Autodesk Inventor part; units mm, degrees
ref_plane "Work Plane7" through (0, -46.7931, -140.1287) normal (0, -0.9797, 0.2004) x (0, -0.2004, -0.9797)
ref_plane "Work Plane8" through (0, 46.7931, -140.1287) normal (0, -0.9797, -0.2004) x (0, 0.2004, -0.9797)
ref_plane "Work Plane9" through (-30, 0, 0) normal (1, 0, 0) x (0, 1, 0)
sketch "Sketch17" plane through (0, 0, 0) normal (1, 0, 0) x (0, 1, 0)
  line L0 (-151.0923, 0) -> (102.6542, 0) construction
  line L1 (0, -220) -> (0, 200)
  circle A0 centre (0, 0) radius 40
  circle A1 centre (0, 0) radius 48.5
  arc A2 (-55.3685, -137.8628) -> (55.3685, -137.8628) centre (0, 54.3203) ccw
  arc A3 (-60, -153.9388) -> (60, -153.9388) centre (0, 140) ccw
  line L2 (55.3685, -137.8628) -> (60, -153.9388)
  line L3 (-60, -153.9388) -> (-55.3685, -137.8628)
  line L4 (-30, -38.1084) -> (-30, -145.6797)
  line L5 (-30, -145.6797) -> (30, -145.6797)
  line L6 (30, -145.6797) -> (30, -38.1084)
  line L7 (-46.7931, -140.1287) -> (-50, -155.804)
  line L8 (46.7931, -140.1287) -> (50, -155.804)
  line L9 (-50, -155.804) -> (-28.8985, -159.3708) construction
  line L10 (-46.7931, -140.1287) -> (-25.9862, -145.1357) construction
  line L11 (-48.3965, -147.9663) -> (-7.733, -156.2855) construction
  arc A4 (26.4209, -129.6797) -> (26, -145.6797) centre (66.4047, -138.7371) ccw
  arc A5 (26.4209, -129.6797) -> (30, -97.6797) centre (-114.8428, -97.6797) ccw
  point P0 (0, -160)
  point P1 (0, -145.6797)
  point P2 (0, -160)
  point P3 (0, -48.5)
  point P4 (0, -145.6797)
  dimension "d173" = 97
  dimension "d174" = 80
  dimension "d224" = 60
  dimension "d229" = 160
  dimension "d230" = 300
  dimension "d231" = 16.7299
  dimension "d232" = 100
  dimension "d233" = 10
  dimension "d235" = 200
  dimension "d241" = 16
  dimension "d242" = 16.7931
  dimension "d243" = 16
  dimension "d244" = 32
  dimension "d245" = 26
sketch "Sketch16" plane through (0, 0, 0) normal (1, 0, 0) x (0, 1, 0)
  circle A0 centre (0, 0) radius 40
  circle A1 centre (0, 0) radius 48.5
  line L0 (0, -201.7) -> (0, 90.2) construction
  line L1 (0, -160) -> (0, -48.5)
  line L2 (30, -38.1084) -> (30, -103.6436)
  line L3 (30, -103.6436) -> (25, -132)
  line L4 (25, -132) -> (50, -132)
  line L5 (50, -132) -> (50, -160)
  line L6 (50, -160) -> (0, -160)
  dimension "d156" = 97
  dimension "d157" = 80
  dimension "d202" = 28
  dimension "d203" = 60
  dimension "d204" = 50
  dimension "d206" = 160
  dimension "d209" = 50
  dimension "d210" = 80
  dimension "d211" = 28.7938
extrude "Extrusion14" [suppressed]
fillet "Fillet10" [suppressed]
mirror "Mirror1" [suppressed]
thicken "Thicken1" [suppressed]
sketch "Sketch19" plane through (0, 0, 0) normal (0, 1, 0) x (-1, 0, 0)
  arc A0 (-110.8458, -111.0605) -> (110.8458, -111.0605) centre (0, -10) ccw
  line L0 (155.1841, 0) -> (-155.1841, 0)
  line L1 (0, -264.129) -> (0, 44.0215)
  line L2 (110.8458, -111.0605) -> (110.8458, -220.1075)
  line L3 (110.8458, -220.1075) -> (-110.8458, -220.1075)
  line L4 (-110.8458, -220.1075) -> (-110.8458, -111.0605)
  point P0 (0, 0)
  point P1 (0, -160)
  point P2 (0, -160)
  point P3 (0, -220.1075)
  dimension "d217" = 150
  dimension "d218" = 0
revolve "Revolution1" [suppressed]
fillet "Fillet15" [suppressed]
revolve "Revolution2" add sketch "Sketch17" angle 360 about axis through (0, 0, -10) along (0, 0, 1) separate body contours L1 L5 L6 A2 L8 A3 | A2 A4 L5 | L8 A2 L2 A3 | A2 L6 L5 A4
ref_plane "Work Plane7" through (0, -46.7931, -140.1287) normal (0, -0.9797, 0.2004) x (0, -0.2004, -0.9797)
split "Split2" plane through (0, -46.7931, -140.1287) removes the side toward (0, -0.9797, 0.2004)
ref_plane "Work Plane8" through (0, 46.7931, -140.1287) normal (0, -0.9797, -0.2004) x (0, 0.2004, -0.9797)
split "Split3" plane through (0, 46.7931, -140.1287) removes the side toward (0, 0.9797, 0.2004)
ref_plane "Work Plane9" through (-30, 0, 0) normal (1, 0, 0) x (0, 1, 0)
split "Split4" plane through (-30, 0, 0) removes the side toward (-1, 0, 0)
ref_plane "Work Plane10" through (30, 0, 0) normal (1, 0, 0) x (0, 1, 0)
split "Split5" plane through (30, 0, 0) removes the side toward (1, 0, 0)
extrude "Extrusion17" add sketch "Sketch17" along normal mid plane 60 contours L1 A1 L6 A5 A4 A2 | A2 A4 L5 | A4 A5 L6 A2 | A2 L6 L5 A4
fillet "Fillet16" radius 5 1 edges at (0, 30, -38.1084)
mirror "Mirror4" about plane through (0, 0, 0) normal (0, 1, 0) of "Extrusion17", "Fillet16"
properties part number "shank_2"
Here's how the part is built. I have some questions about the finished solid (model axes, mm). Round coordinates to 2 decimals unless told otherwise and drop trailing zeros. Order: outer loops, then holes, each group sorted by start corner. A loop starts at its lowest first (then second) coordinate and runs counter-clockwise, first axis right, second up. Notation, with made-up numbers: M 49.5,34 L 54.5,34 A19 ccw 54.5,38 Z; hole C 0,21.5 d3. An arc over 180 degrees is marked long. Use CSV: the item, a comma, the result in double quotes.
1) If we mould it in two halves opening along Y, with no side actions, what happens to faces 1 (the flat face through (-30, -1, -100)), 2 (the cylindrical face through (-0.42, 27.52, -42.98)), 3 (the flat face through (-0.42, 48.144, -146.732))? For each: pulls with the +Y half, pulls with the -Y half, needs draft (parallel to the pull), parting line crosses it, or undercut.
Taken from the geometry:
face 1,"needs draft"
face 2,"undercut"
face 3,"pulls with the +Y half"
2) I want a section at A-A (x = 18). List the corners of the cut face in (y, z) for me, then the cut area to 3 significant figures.
Taken from the geometry:
outline,"M -49.89,-155.27 A299.46 ccw 49.89,-155.27 L 46.63,-139.33 A199.19 cw 30,-142.6 L 30,-47.3 A5 ccw 22.66,-42.88 A48.5 cw -22.66,-42.88 A5 ccw -30,-47.3 L -30,-142.6 A199.19 cw -46.63,-139.33 Z"
area,"7,370 mm^2"
3) I need wall thicknesses on line 1 along Y through (x, z) = (14.5, -94); line 2 along Z through (x, y) = (-12.5, -6); line 3 along Z through (x, y) = (5.5, 43). Which ranges of each line are inside material? Lowest first, please. Write a range as [from, to].
Taken from the geometry:
line 1,"[-30, 30]"
line 2,"[-159.68, -48.13]"
line 3,"[-156.85, -140.93]"
4) I want a section at B-B (z = -107.5). List the corners of the cut face in (x, y) for me.
Taken from the geometry:
outline,"M -30,-30 L 30,-30 L 30,30 L -30,30 Z"
5) I want a section at D-D (x = -17). List the corners of the cut face in (y, z) for me.
Taken from the geometry:
outline,"M -49.9,-155.33 A299.52 ccw 49.9,-155.33 L 46.65,-139.42 A199.28 cw 30,-142.68 L 30,-47.3 A5 ccw 22.66,-42.88 A48.5 cw -22.66,-42.88 A5 ccw -30,-47.3 L -30,-142.68 A199.28 cw -46.65,-139.42 Z"
6) I'm going to push flat-ended pins straight in: P1, Ø6, axis at x = 18, y = 37.5, coming from the +Z side; P2, Ø1.5, axis at x = -15, y = -13, coming from the +Z side; P3, Ø1, axis at x = 10.5, z = -93.5, coming from the +Y side. Where does each tip first touch, or does it pass through?
Taken from the geometry:
P1,"z = -140.64"
P2,"z = -46.51"
P3,"y = 30"
7) I want a section at C-C (y = 19). List the corners of the cut face in (x, z) for me.
Taken from the geometry:
outline,"M -30,-157.89 A299.4 ccw 30,-157.89 L 30,-44.62 L -30,-44.62 Z"
